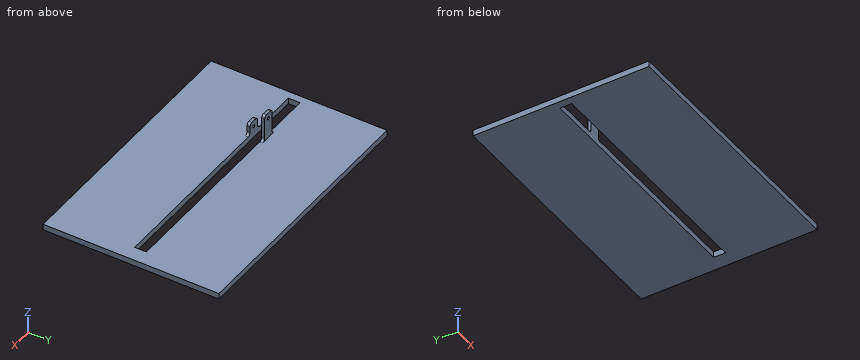
from build123d import *

# Parameters (mm, degrees)
SKETCH1_W           = 1300
SKETCH1_H           = 600
SKETCH1_W_2         = 1117.676372874
SKETCH1_H_2         = 40
BOSS_EXTRUDE1_DEPTH = 20
SKETCH2_W           = 40
SKETCH2_H           = 10
BOSS_EXTRUDE2_DEPTH = 40
SKETCH3_R           = 5
CUT_EXTRUDE1_DEPTH  = 10
SKETCH4_W           = 40
SKETCH4_H           = 10
BOSS_EXTRUDE3_DEPTH = 50
SKETCH5_R           = 5
CUT_EXTRUDE2_DEPTH  = 10
FILLET1_R           = 10
FILLET2_R           = 10
FILLET3_R           = 10
FILLET4_R           = 10
FILLET5_R           = 10
FILLET6_R           = 10
FILLET7_R           = 10
FILLET8_R           = 10
SKETCH6_W           = 20
SKETCH6_H           = 40
BOSS_EXTRUDE4_DEPTH = 260
SKETCH7_W           = 20
SKETCH7_H           = 40
BOSS_EXTRUDE5_DEPTH = 35
SKETCH8_W           = 20
SKETCH8_H           = 600
CUT_EXTRUDE3_DEPTH  = 100
SKETCH9_W           = 20
SKETCH9_H           = 600
CUT_EXTRUDE4_DEPTH  = 300


with BuildPart() as part:
    # Sketch1 → Boss-Extrude1 (new body)
    with BuildSketch(Plane.XY):
        Rectangle(SKETCH1_W, SKETCH1_H)
        Rectangle(SKETCH1_W_2, SKETCH1_H_2, mode=Mode.SUBTRACT)
    extrude(amount=BOSS_EXTRUDE1_DEPTH)

    # Sketch2 → Boss-Extrude2 (add)
    with BuildSketch(Plane.XY.offset(20)):
        with Locations((-338.838186437, 25)):
            Rectangle(SKETCH2_W, SKETCH2_H)
        with Locations((-338.838186437, -25)):
            Rectangle(SKETCH2_W, SKETCH2_H)
    extrude(amount=BOSS_EXTRUDE2_DEPTH)

    # Sketch3 → Cut-Extrude1 (cut)
    with BuildSketch(Plane.XZ.offset(30)):
        with Locations((-338.838186437, 40)):
            Circle(SKETCH3_R)
    extrude(amount=-CUT_EXTRUDE1_DEPTH, mode=Mode.SUBTRACT)

    # Sketch4 → Boss-Extrude3 (add)
    with BuildSketch(Plane.XY.offset(60)):
        with Locations((-338.838186437, 25)):
            Rectangle(SKETCH4_W, SKETCH4_H)
    extrude(amount=BOSS_EXTRUDE3_DEPTH)

    # Sketch5 → Cut-Extrude2 (cut)
    with BuildSketch(Plane.XZ.offset(-20)):
        with Locations(Location((-338.838186437, 90, 0), (0, 0, 270))):
            Circle(SKETCH5_R)
    extrude(amount=-CUT_EXTRUDE2_DEPTH, mode=Mode.SUBTRACT)

    # Fillet1
    fillet1_edges = [part.edges().sort_by_distance(p)[0] for p in [
        (-318.838186437, -25, 20),
    ]]
    fillet(fillet1_edges, radius=FILLET1_R)

    # Fillet2
    fillet2_edges = [part.edges().sort_by_distance(p)[0] for p in [
        (-318.838186437, 25, 20),
    ]]
    fillet(fillet2_edges, radius=FILLET2_R)

    # Fillet3
    fillet3_edges = [part.edges().sort_by_distance(p)[0] for p in [
        (-358.838186437, -25, 20),
    ]]
    fillet(fillet3_edges, radius=FILLET3_R)

    # Fillet4
    fillet4_edges = [part.edges().sort_by_distance(p)[0] for p in [
        (-358.838186437, 25, 20),
    ]]
    fillet(fillet4_edges, radius=FILLET4_R)

    # Fillet5
    fillet5_edges = [part.edges().sort_by_distance(p)[0] for p in [
        (-318.838186437, -25, 60),
    ]]
    fillet(fillet5_edges, radius=FILLET5_R)

    # Fillet6
    fillet6_edges = [part.edges().sort_by_distance(p)[0] for p in [
        (-358.838186437, -25, 60),
    ]]
    fillet(fillet6_edges, radius=FILLET6_R)

    # Fillet7
    fillet7_edges = [part.edges().sort_by_distance(p)[0] for p in [
        (-358.838186437, 25, 110),
    ]]
    fillet(fillet7_edges, radius=FILLET7_R)

    # Fillet8
    fillet8_edges = [part.edges().sort_by_distance(p)[0] for p in [
        (-318.838186437, 25, 110),
    ]]
    fillet(fillet8_edges, radius=FILLET8_R)

    # Sketch6 → Boss-Extrude4 (add)
    with BuildSketch(Plane.ZY.offset(-558.838186437)):
        with Locations((10, 0)):
            Rectangle(SKETCH6_W, SKETCH6_H)
    extrude(amount=BOSS_EXTRUDE4_DEPTH)

    # Sketch7 → Boss-Extrude5 (add)
    with BuildSketch(Plane(origin=(-558.838186437, 0, 0), x_dir=(0, 0, -1), z_dir=(1, 0, 0))):
        with Locations((-10, 0)):
            Rectangle(SKETCH7_W, SKETCH7_H)
    extrude(amount=BOSS_EXTRUDE5_DEPTH)

    # Sketch8 → Cut-Extrude3 (cut)
    with BuildSketch(Plane.ZY.offset(650)):
        with Locations((10, 0)):
            Rectangle(SKETCH8_W, SKETCH8_H)
    extrude(amount=-CUT_EXTRUDE3_DEPTH, mode=Mode.SUBTRACT)

    # Sketch9 → Cut-Extrude4 (cut)
    with BuildSketch(Plane(origin=(650, 0, 0), x_dir=(0, 0, -1), z_dir=(1, 0, 0))):
        with Locations((-10, 0)):
            Rectangle(SKETCH9_W, SKETCH9_H)
    extrude(amount=-CUT_EXTRUDE4_DEPTH, mode=Mode.SUBTRACT)


solid = part.part
Here's how the part is built. I have some questions about the finished solid (model axes, mm). Round coordinates to 2 decimals unless told otherwise and drop trailing zeros. Order: outer loops, then holes, each group sorted by start corner. A loop starts at its lowest first (then second) coordinate and runs counter-clockwise, first axis right, second up. Notation, with made-up numbers: M 54,-18 L 112,-18 A20 cw 112,-9 Z; hole C 51.25,-15.75 d1. An arc over 180 degrees is marked long. Return JSON: item names as keys, results as strings. Group by question number.
1. Please list where these lines run through material, in increasing order: probe 1 along X at (y, z) = (24, 90); probe 2 along Y at (x, z) = (158, 11.5); probe 3 along Z at (x, y) = (124, 67).
2. If we section it at C-C on z = 70.5: List the corners of the cut face in (x, y) for me.
3. If we section it at B-B on y = -128: List the corners of the cut face in (x, z) for me, then the cut area to 3 significant figures.
4. I'm going to push flat-ended pins straight in: pin 1 Ø8 at (y, z) = (23.5, 63) entering from -X; pin 2 Ø11 at (x, y) = (-334, -27) entering from +Z; pin 3 Ø6 at (x, z) = (-338.84, 40) entering from +Y; pin 4 Ø8 at (x, z) = (-338.84, 90) entering from -Y. Where does each tip first touch, or does it pass through?
5. If we section it at A-A on x = -203.5: List the corners of the cut face in (y, z) for me.
Reply:
{
 "1": {"probe 1": "-358.84 to -343.84, -333.84 to -318.84", "probe 2": "-300 to -20, 20 to 300", "probe 3": "0 to 20"},
 "2": {"outline": "M -358.84,20 L -318.84,20 L -318.84,30 L -358.84,30 Z"},
 "3": {"outline": "M -550,0 L 350,0 L 350,20 L -550,20 Z", "area": "18,000 mm^2"},
 "4": {"pin 1": "x = -358.84", "pin 2": "z = 60", "pin 3": "y = 30", "pin 4": "through"},
 "5": {"outline": "M -300,0 L -20,0 L -20,20 L -300,20 Z; M 20,0 L 300,0 L 300,20 L 20,20 Z"}
}
